from build123d import *

# Parameters (mm, degrees)
SALIENTE_EXTRUIR1_DEPTH = 215.9
VACIADO2_T              = -2
CROQUIS2_W              = 55
CROQUIS2_H              = 171.9
CORTAR_EXTRUIR1_DEPTH   = 215.9
CROQUIS3_W              = 55
CROQUIS3_H              = 172.561085537
CORTAR_EXTRUIR2_DEPTH   = 215.9
CROQUIS4_W              = 55.15393927
CROQUIS4_H              = 171.9
CORTAR_EXTRUIR3_DEPTH   = 215.9


with BuildPart() as part:
    # Croquis1 → Saliente-Extruir1 (new body)
    with BuildSketch(Plane(origin=(0, 0, 0), x_dir=(1, 0, 0), z_dir=(0, 1, 0))):
        Polygon((-87, 2.4695933), (-45.638730535, -74.109413479), (41.361269465, -76.579006779), (87, -2.4695933), (45.638730535, 74.109413479), (-41.361269465, 76.579006779), align=None)
    extrude(amount=-SALIENTE_EXTRUIR1_DEPTH)

    # Vaciado2
    vaciado2_openings = [part.faces().sort_by_distance(p)[0] for p in [
        (0, 0, 0),
    ]]
    offset(amount=VACIADO2_T, openings=vaciado2_openings, kind=Kind.INTERSECTION)

    # Croquis2 → Cortar-Extruir1 (cut)
    with BuildSketch(Plane(origin=(-2.138730535, 0, 75.344210129), x_dir=(0.9995973571275039, 0, 0.02837470041620955), z_dir=(-0.02837470041620955, 0, 0.9995973571275039))):
        with Locations((0, -107.95)):
            Rectangle(CROQUIS2_W, CROQUIS2_H)
    extrude(amount=-CORTAR_EXTRUIR1_DEPTH, mode=Mode.SUBTRACT)

    # Croquis3 → Cortar-Extruir2 (cut)
    with BuildSketch(Plane(origin=(64.180634732, 0, 39.52430004), x_dir=(0.5243718899489567, 0, -0.8514893546201029), z_dir=(0.8514893546201029, 0, 0.5243718899489567))):
        with Locations((0, -107.619457232)):
            Rectangle(CROQUIS3_W, CROQUIS3_H)
    extrude(amount=-CORTAR_EXTRUIR2_DEPTH, mode=Mode.SUBTRACT)

    # Croquis4 → Cortar-Extruir3 (cut)
    with BuildSketch(Plane(origin=(66.319365268, 0, -35.819910089), x_dir=(-0.47522546717854747, 0, -0.8798640550363058), z_dir=(0.8798640550363059, 0, -0.4752254671785475))):
        with Locations((-1.247199632, -107.95)):
            Rectangle(CROQUIS4_W, CROQUIS4_H)
    extrude(amount=-CORTAR_EXTRUIR3_DEPTH, mode=Mode.SUBTRACT)


solid = part.part
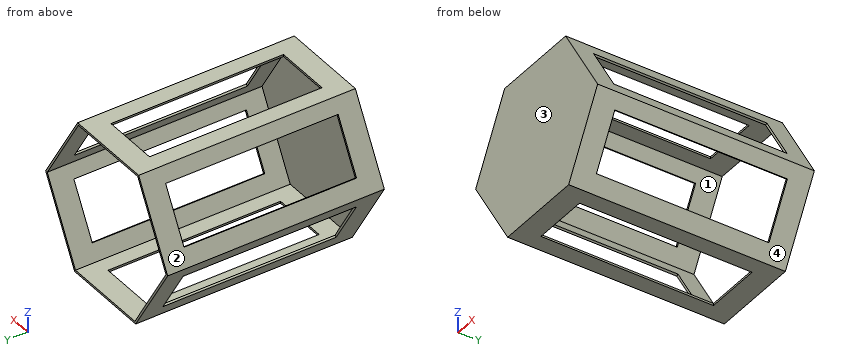
The listing builds one solid part. Answer for the finished solid, in the listing's coordinates (mm). Face numbers are marked on the shaded views. Give positions to 0.01 mm unless a question says otherwise; leave off trailing zeros. Loops run counter-clockwise (first coordinate to the right, second up) from the corner with the lowest first, then second, coordinate; pieces in that order, holes last. Notation, with made-up numbers: M 17,8.25 L 25,8.25 A10 cw 25,22.25 Z; hole C 74,7 d4. An arc over 180 degrees is marked long. Answer as CSV lines item,"result".
Item 1: Straight lines are drawn through the part: line 1 along Y through (x, z) = (-59.5, -44.5); line 2 along Y through (x, z) = (-61.5, -28); line 3 along Z through (x, y) = (-42, -28). For each, find the intervals that lie inside material, in ascending order. Write a range as [from, to].
Values follow:
line 1,"y = [-215.9, -193.9], [-21.34, 0]"
line 2,"y = [-215.9, -213.9]"
line 3,"z = [-75.54, -71.73], [72.21, 74.21]"
Item 2: The mould has two halves that part along Z. Classify the marked faces 1, 2, 3 and 4: released by +Z, released by -Z, zero draft, split by the parting line, or undercut.
Values follow:
face 1,"undercut"
face 2,"released by +Z"
face 3,"zero draft"
face 4,"released by -Z"
Item 3: The part is cut by section B-B (x = 22). Give the vertices of the cut face in (y, z), and give its area (3 significant figures).
Values follow:
outline,"M -215.9,-74.78 L -193.9,-74.78 L -193.9,-72.78 L -213.9,-72.78 L -213.9,74.03 L -193.9,74.03 L -193.9,76.03 L -215.9,76.03 Z; M -22,-74.78 L 0,-74.78 L 0,-72.78 L -22,-72.78 Z; M -22,74.03 L 0,74.03 L 0,76.03 L -22,76.03 Z"
area,"470 mm^2"
Item 4: The part is cut by section A-A (z = -50). Give the vertices of the cut face in (x, y), and give its area (3 significant figures).
Values follow:
outline,"M -57.73,-215.9 L 58.66,-215.9 L 58.66,-193.9 L 56.39,-193.9 L 56.39,-213.9 L -55.38,-213.9 L -55.38,-193.9 L -57.73,-193.9 Z; M -57.73,-21.34 L -55.38,-21.34 L -55.38,0 L -57.73,0 Z; M 56.39,-22 L 58.66,-22 L 58.66,0 L 56.39,0 Z"
area,"425 mm^2"
Item 5: The part is cut by section D-D (z = 7). Give the vertices of the cut face in (x, y).
Values follow:
outline,"M -81.89,-215.9 L 84.21,-215.9 L 84.21,0 L 81.86,0 L 81.86,-213.9 L -79.61,-213.9 L -79.61,0 L -81.89,0 Z"
Item 6: Given pin 1 Ø5 at (y, z) = (-42.5, -12) entering from +X; pin 2 Ø8 at (y, z) = (-59, -7) entering from +X; pin 3 Ø1.5 at (y, z) = (-44.5, -6) entering from -X; pin 4 Ø1.5 at (x, y) = (-54.5, -109) entering from +Z, each flat-ended and moving along its own axis, determine where each tip first touches the part or whether it passes through.
Values follow:
pin 1,"stops at x = 80.54"
pin 2,"stops at x = 84.05"
pin 3,"stops at x = -85.29"
pin 4,"passes through"
Item 7: The part is cut by section C-C (y = -177.5). Give the number of separate pieces and of enclosed holes in the cut face, and give its area (3 significant figures).
Values follow:
separate pieces,"6"
enclosed holes,"0"
area,"370 mm^2"
